Can you work these out from the model? Positions are in its coordinate system, mm. A direction names the side the tool comes from. Give positions to 0.01 mm unless a question says otherwise; leave off trailing zeros. Order: outer loops, then holes, each group sorted by start corner. A loop starts at its lowest first (then second) coordinate and runs counter-clockwise, first axis right, second up.
Item 1: Which directions (+Z, -Z, +X, -X, +Y, -Y) give clear straight access to the entire face, cutting with the end or side of a thin tool? Please do faces 4 (the flat face through (44.45, 2, -2)), 5 (the cylindrical face through (12.52, 0.69, -3.1)), 6 (the cylindrical face through (28.53, -17.59, -17.32)).
Item 2: If we mould it in two halves opening along Y, with no side actions, what happens to faces 1 (the flat face through (0, 11, 1)), 2 (the cylindrical face through (12.522, -11.012, -49.592)), 3 (the flat face through (25.4, 0, 0))? For each: +Y half, -Y half, draft (parallel to the pull), parting line (faces both ways), or undercut.
Item 3: I want a section at A-A, the plane x = 11. Write out the boundary of the cut face in (y, z) (3 decimals), then the cut area to 3 significant figures.
Item 4: If I drill on line 1 along Z through (x, y) = (13, 0) (3 decimals); line 2 along X through (y, z) = (-6, 42.5); line 3 along Y through (x, z) = (13, 5.5), over which ranges is the centre line in solid material (lowest first)?
Item 5: I'm going to push flat-ended pins straight in: pin 1 Ø5 at (x, z) = (24, -1.5) entering from -Y; pin 2 Ø1 at (x, z) = (20, 9) entering from +Y; pin 3 Ø6 at (x, z) = (14.5, -11) entering from +Y; pin 4 Ø1.5 at (x, z) = (12, -1) entering from +Y. Where does each tip first touch, or does it pass through?
```python
from build123d import *

# Parameters (mm, degrees)
F0_R     = 50.8
F1_DEPTH = 25.4
F3_D     = 6.35
F4_R     = 25.4
F5_DEPTH = 19.05
F6_R     = 12.7


with BuildPart() as f1:
    # F0 (on Right) → F1 (new body)
    with BuildSketch(Plane.YZ):
        Circle(F0_R)
    extrude(amount=F1_DEPTH)

    # F3 (through all)
    with Locations(Plane.YZ.offset(25.4)):
        with Locations((0, 0)):
            Hole(F3_D / 2)

    # F4 (on face) → F5 (join)
    with BuildSketch(Plane.YZ.offset(25.4)):
        with Locations((2.568165, -1.866857)):
            Circle(F4_R)
    extrude(amount=F5_DEPTH)

    # F6
    f6_edges = [f1.edges().sort_by_distance(p)[0] for p in [
        (44.45, -22.831835, -1.866857),
    ]]
    fillet(f6_edges, radius=F6_R)


solid = f1.part
```
Results list:
1. face 4: +Z, -Z, +X, +Y, -Y
1. face 5: -X
1. face 6: +X
2. face 1: draft
2. face 2: parting line
2. face 3: undercut
3. outline: circle Ø101.6 at (0, 0); hole circle Ø6.35 at (0, 0)
3. area: 8,080 mm2
4. line 1: z = -50.8 to -3.175, 3.175 to 50.8
4. line 2: x = 0 to 25.4
4. line 3: y = -50.5 to 50.5
5. pin 1: stops at y = -50.8
5. pin 2: stops at y = 50.08
5. pin 3: stops at y = 50.17
5. pin 4: stops at y = 50.8
